Study the drawing (mm; zero at the part's minimum x, y, z) and answer. A direction names the side the tool comes from. Give positions to 0.01 mm unless a question says otherwise; leave off trailing zeros. Order: outer loops, then holes, each group sorted by start corner. A loop starts at its lowest first (then second) coordinate and runs counter-clockwise, first axis right, second up.
Item 1: A cutting plane is placed at D-D (x = 64). Write down the section's boundary in (y, z) (1 decimal), plus the area to 3 significant figures.
Item 2: Given pin 1 Ø2 at (x, y) = (43.5, 49) entering from -Z (1 decimal); pin 2 Ø20.5 at (y, z) = (42.5, 14) entering from -X; pin 3 Ø2 at (x, y) = (67, 33.5) entering from +Z; pin 4 Ø8 at (x, z) = (28.5, 11) entering from +Y, each flat-ended and moving along its own axis, determine where each tip first touches the part or whether it passes through.
Item 3: A cutting plane is placed at B-B (z = 33). Write down the section's boundary in (x, y), plus the area to 3 significant figures.
Item 4: A cutting plane is placed at C-C (y = 41.5). Write down the section's boundary in (x, z) (1 decimal).
Item 5: The mould has two halves that part along Z. Classify the marked faces 5, 6, 7 and 8: +Z half, -Z half, draft (parallel to the pull), parting line (faces both ways), or undercut.
Item 6: Find the intervals of material crossed by line 1 along X through (y, z) = (16.5, 4.5); line 2 along Y through (x, z) = (36.5, 30.5); line 3 along Z through (x, y) = (71, 47.5) (1 decimal), in increasing order.
Item 7: A cutting plane is placed at A-A (x = 40.5). Write down the section's boundary in (y, z) (1 decimal).
Item 8: Which of the six approach directions +Z, -Z, +X, -X, +Y, -Y give full straight-line access (tool end or side, diameter ignored) to the marked faces 1, 2, 3 and 4?
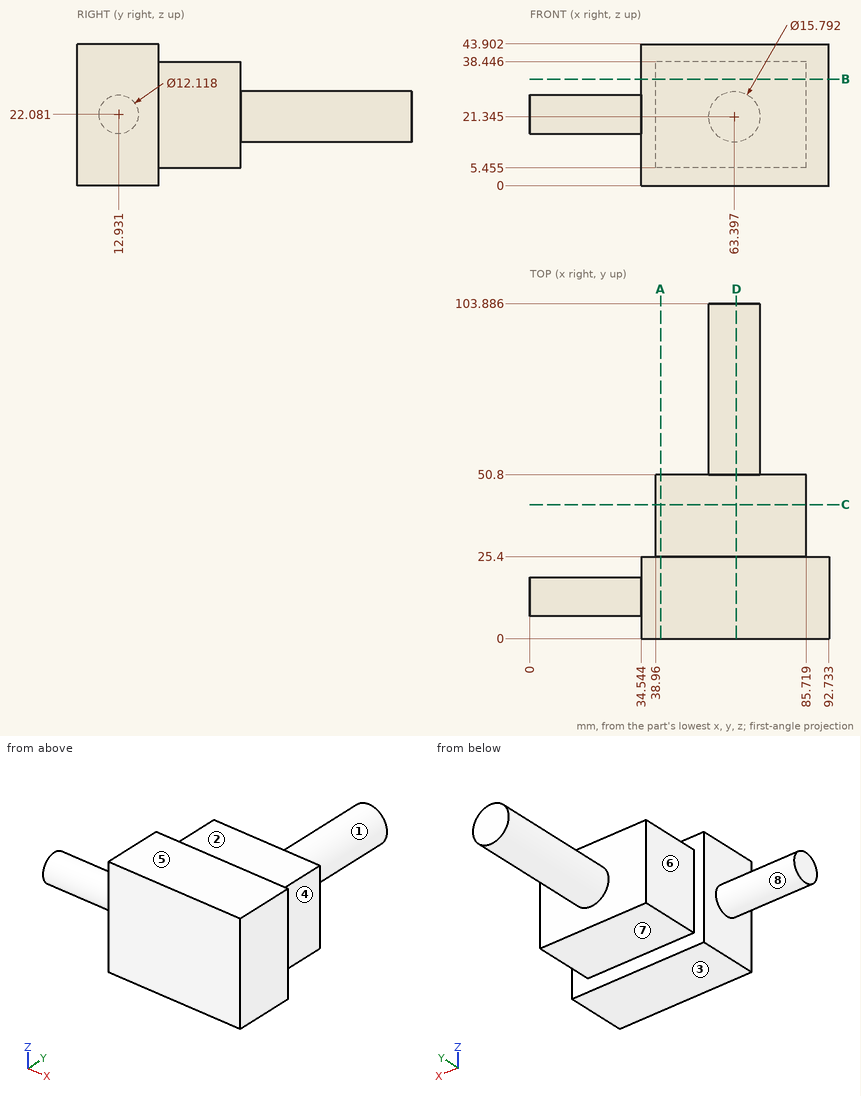
Response values:
1. outline: (0, 0) - (25.4, 0) - (25.4, 5.5) - (50.8, 5.5) - (50.8, 13.5) - (103.9, 13.5) - (103.9, 29.2) - (50.8, 29.2) - (50.8, 38.4) - (25.4, 38.4) - (25.4, 43.9) - (0, 43.9) - close
1. area: 2,790 mm2
2. pin 1: stops at z = 5.5
2. pin 2: stops at x = 38.96
2. pin 3: stops at z = 38.45
2. pin 4: passes through
3. outline: (34.54, 0) - (92.73, 0) - (92.73, 25.4) - (85.72, 25.4) - (85.72, 50.8) - (38.96, 50.8) - (38.96, 25.4) - (34.54, 25.4) - close
3. area: 2,670 mm2
4. outline: (39, 5.5) - (85.7, 5.5) - (85.7, 38.4) - (39, 38.4) - close
5. face 5: +Z half
5. face 6: draft
5. face 7: -Z half
5. face 8: parting line
6. line 1: x = 34.54 to 92.73
6. line 2: y = 0 to 25.4
6. line 3: z = 5.5 to 38.4
7. outline: (0, 0) - (25.4, 0) - (25.4, 5.5) - (50.8, 5.5) - (50.8, 38.4) - (25.4, 38.4) - (25.4, 43.9) - (0, 43.9) - close
8. face 1: +Y
8. face 2: +Z, +X, -X, +Y
8. face 3: -Z, +X, -X, +Y, -Y
8. face 4: +Z, -Z, +X, +Y
